Autodesk Inventor part; units mm, degrees
ref_plane "YZ Plane" through (0, 0, 0) normal (1, 0, 0) x (0, 1, 0)
ref_plane "XZ Plane" through (0, 0, 0) normal (0, 1, 0) x (-1, 0, 0)
ref_plane "XY Plane" through (0, 0, 0) normal (0, 0, 1) x (1, 0, 0)
sketch "Boceto1" plane through (0, 0, 0) normal (0, 0, 1) x (1, 0, 0)
  line L0 (0, 0) -> (50, 0)
  line L1 (50, 0) -> (50, 50)
  line L2 (50, 50) -> (0, 50)
  line L3 (0, 50) -> (0, 0)
  line L4 (50, 0) -> (0, 0)
  line L5 (0, 0) -> (0, 10)
  line L6 (0, 10) -> (50, 10)
  line L7 (50, 10) -> (50, 0)
  dimension "d0" = 50
  dimension "d1" = 50
  dimension "d2" = 10
extrude "Extrusión1" add sketch "Boceto1" along normal blind 10
sketch "Boceto2" plane through (0, 0, 10) normal (0, 0, 1) x (1, 0, 0)
  line L0 (0, 0) -> (50, 0)
  line L1 (0, 50) -> (0, 0)
  line L2 (50, 0) -> (0, 0)
  line L3 (0, 0) -> (0, 10)
  line L4 (0, 10) -> (50, 10)
  line L5 (50, 10) -> (50, 0)
  dimension "d5" = 10
extrude "Extrusión2" add sketch "Boceto2" along normal blind 30
sketch "Boceto3" plane through (0, 0, 10) normal (0, 0, 1) x (1, 0, 0)
  circle A0 centre (25, 25) radius 3.4
  line L0 (0, 50) -> (0, 10)
  line L1 (0, 0) -> (50, 0)
  dimension "d8" = 6.8
  dimension "d9" = 25
  dimension "d10" = 25
extrude "Extrusión3" cut sketch "Boceto3" against normal blind 10
sketch "Boceto4" plane through (0, 10, 10) normal (0, 1, 0) x (1, 0, 0)
  circle A0 centre (25, -20) radius 5.1
  line L0 (50, 10) -> (0, 10)
  line L1 (0, 0) -> (0, -30)
  dimension "d13" = 10.2
  dimension "d14" = 30
  dimension "d15" = 25
extrude "Extrusión4" cut sketch "Boceto4" against normal blind 10
sketch "Boceto5" plane through (0, 0, 0) normal (-1, 0, 0) x (0, 0, 1)
  line L0 (0, 50) -> (10, 50)
  line L1 (10, 10) -> (40, 10)
  line L2 (10, 50) -> (40, 10)
  line L3 (40, 10) -> (10, 10)
  line L4 (10, 10) -> (10, 50)
  line L5 (10, 50) -> (10, 10)
  point P0 (0, 0)
extrude "Extrusión5" add sketch "Boceto5" against normal blind 5
sketch "Boceto6" plane through (50, 0, 0) normal (1, 0, 0) x (0, 0, -1)
  line L0 (-10, 50) -> (-40, 10)
  line L1 (-10, 10) -> (-40, 10)
  line L2 (-10, 50) -> (-40, 10)
  line L3 (-40, 10) -> (-10, 10)
  line L4 (-10, 50) -> (-10, 10)
  line L5 (-10, 10) -> (-10, 50)
  point P0 (0, 0)
sketch "Boceto7" plane through (50, 0, 0) normal (1, 0, 0) x (0, 0, -1)
  point P0 (0, 0)
sketch "Boceto8" plane through (0, 0, 10) normal (0, 0, 1) x (1, 0, 0)
  point P0 (0, 0)
extrude "Extrusión6" add sketch "Boceto6" against normal blind 5
sketch "Boceto9" plane through (0, 0, 0) normal (0, 0, -1) x (-1, 0, 0)
  line L0 (-5, 5) -> (-45, 5)
  line L1 (-45, 5) -> (-45, 45)
  line L2 (-45, 45) -> (-5, 45)
  line L3 (-5, 45) -> (-5, 5)
  line L4 (-50, 0) -> (-50, 50)
  line L5 (-50, 50) -> (0, 50)
  line L6 (0, 50) -> (0, 0)
  line L7 (0, 0) -> (-50, 0)
  line L8 (-50, 0) -> (-50, 50)
  line L9 (-50, 50) -> (0, 50)
  line L10 (0, 50) -> (0, 0)
extrude "Extrusión7" add sketch "Boceto9" along normal blind 20
sketch "Boceto10" plane through (50, 0, 40) normal (1, 0, 0) x (0, 0, -1)
  line L0 (0, 0) -> (0, 10)
  circle A0 centre (50, 25) radius 3.375
  line L1 (60, 0) -> (0, 0)
  line L2 (60, 50) -> (60, 0)
  point P0 (40, 0)
  dimension "d28" = 40
  dimension "d29" = 6.75
sketch "Boceto12" plane through (0, 0, 40) normal (-1, 0, 0) x (0, 0, 1)
  circle A0 centre (-50, 25) radius 3.375
  line L0 (-60, 0) -> (-60, 50)
  line L1 (-30, 50) -> (-60, 50)
  point P0 (-40, 0)
  dimension "d35" = 6.75
extrude "Extrusión9" cut sketch "Boceto10" against normal blind 5
extrude "Extrusión11" cut sketch "Boceto12" against normal blind 5
properties part number "UnionLlantaOmega2" material "Plástico ABS"
For this review, take the finished solid that the model builds, in its own axes (mm). A direction names the side the tool comes from. Give positions to 0.01 mm unless a question says otherwise; leave off trailing zeros. Write each loop counter-clockwise with the first axis right and the second up, starting at its lowest first coordinate (ties: lowest second). Pieces come first, ordered by that corner, then holes. Notation, with made-up numbers: M 63,-7 L 83,-7 A20 ccw 83,27 Z; hole C 42,62 d1. An arc over 180 degrees is marked long. One line per item, written item: value.
1) Take a section at C-C, the plane y = 7. Write out the cut boundary in (x, z), then the cut area to 3 significant figures.
Results are:
outline: M 0,-20 L 5,-20 L 5,0 L 45,0 L 45,-20 L 50,-20 L 50,40 L 0,40 Z; hole C 25,30 d10.2
area: 2,120 mm²
2) For faces 1 (the flat face through (25, 5, -10)), 2 (the flat face through (25, 50, -5)), 3 (the flat face through (5, 21, 18)), list the 3-axis set-ups (+Z, -Z, +X, -X, +Y, -Y) from which the entire face can be reached by the end or side of a thin tool; tool diameter is ignored.
Results are:
face 1: -Z
face 2: +Z, -Z, +X, -X, +Y
face 3: +Z, +Y
3) For P1, Ø6, axis at x = 25, y = 25, coming from the -Z side; P2, Ø2, axis at x = 36, y = 38, coming from the -Z side; P3, Ø5, axis at y = 23, z = 9.5, coming from the -X side; P4, Ø9, axis at x = 33, z = 21.5, coming from the +Y side, all flat-tipped, find the tip position at first contact; note any pin that passes through.
Results are:
P1: passes through
P2: stops at z = 0
P3: stops at x = 0
P4: stops at y = 10
4) Take a section at B-B, the plane z = -10. Write out the cut boundary in (x, y) (3 decimals).
Results are:
outline: M 0,0 L 50,0 L 50,21.625 L 45,21.625 L 45,5 L 5,5 L 5,21.625 L 0,21.625 Z; M 0,28.375 L 5,28.375 L 5,45 L 45,45 L 45,28.375 L 50,28.375 L 50,50 L 0,50 Z
5) Take a section at A-A, the plane x = 25. Write out the cut boundary in (y, z), then the cut area to 3 significant figures.
Results are:
outline: M 0,-20 L 5,-20 L 5,0 L 21.6,0 L 21.6,10 L 10,10 L 10,24.9 L 0,24.9 Z; M 0,35.1 L 10,35.1 L 10,40 L 0,40 Z; M 28.4,0 L 45,0 L 45,-20 L 50,-20 L 50,10 L 28.4,10 Z
area: 830 mm²
6) Take a section at D-D, the plane z = -3. Write out the cut boundary in (x, y), then the cut area to 3 significant figures.
Results are:
outline: M 0,0 L 50,0 L 50,50 L 0,50 Z; hole M 5,5 L 45,5 L 45,45 L 5,45 Z
area: 900 mm²
7) For line 1 (Y direction, x = 20, z = -14.5); line 2 (Y direction, x = 47.8, z = -10) (3 decimals), list the stretches that pass through material, from the lowest coordinate up. Write a range as from..to.
Results are:
line 1: y = 0..5, 45..50
line 2: y = 0..21.625, 28.375..50
8) The part is to be moulded in two halves that separate along Z. For faces 4 (the flat face through (25, 5, 40)), 5 (the cylindrical face through (2.46, 25.15, -13.37)), 6 (the flat face through (25, 45, -10)), say which applies: +Z half, -Z half, draft (parallel to the pull), parting line (faces both ways), or undercut.
Results are:
face 4: +Z half
face 5: undercut
face 6: draft
